Input: part model. Units: mm. Frame: model coordinates. A direction names the side the tool comes from. Coordinates: 2 decimals unless noted, no trailing zeros. Loops run counter-clockwise (first coordinate to the right, second up) from the corner with the lowest first, then second, coordinate; pieces in that order, holes last.
```python
from build123d import *

# Parameters (mm, degrees)
SKETCH1_W           = 350
SKETCH1_H           = 150
BOSS_EXTRUDE1_DEPTH = 10
SKETCH2_W           = 328
SKETCH2_H           = 126
SKETCH2_W_2         = 70
SKETCH2_H_2         = 110
SKETCH2_W_3         = 27.5
SKETCH2_H_3         = 55
CUT_EXTRUDE1_DEPTH  = 9.5


with BuildPart() as part:
    # Sketch1 → Boss-Extrude1 (new body)
    with BuildSketch(Plane(origin=(0, 0, 0), x_dir=(1, 0, 0), z_dir=(0, 1, 0))):
        Rectangle(SKETCH1_W, SKETCH1_H)
    extrude(amount=BOSS_EXTRUDE1_DEPTH)

    # Sketch2 → Cut-Extrude1 (cut)
    # profile 1 of 5: a face of its own
    with BuildSketch(Plane(origin=(0, 10, 0), x_dir=(1, 0, 0), z_dir=(0, 1, 0))):
        with Locations((-1, -2)):
            Rectangle(SKETCH2_W, SKETCH2_H)
        with Locations((-122, -2)):
            Rectangle(SKETCH2_W_2, SKETCH2_H_2, mode=Mode.SUBTRACT)
        with Locations((-41, -2)):
            Rectangle(SKETCH2_W_2, SKETCH2_H_2, mode=Mode.SUBTRACT)
        with Locations((40, -2)):
            Rectangle(SKETCH2_W_2, SKETCH2_H_2, mode=Mode.SUBTRACT)
        with Locations((121, -2)):
            Rectangle(SKETCH2_W_2, SKETCH2_H_2, mode=Mode.SUBTRACT)
    # profile 2 of 5: a face of its own
    with BuildSketch(Plane(origin=(0, 10, 0), x_dir=(1, 0, 0), z_dir=(0, 1, 0))):
        with BuildLine():
            Line((-147, -44.243757332), (-147, 40.243757332))
            ThreePointArc((-147, 40.243757332), (-147.353553391, 43.353553391), (-144.243757332, 43))
            Line((-144.243757332, 43), (-99.756242668, 43))
            ThreePointArc((-99.756242668, 43), (-96.646446609, 43.353553391), (-97, 40.243757332))
            Line((-97, 40.243757332), (-97, -44.243757332))
            ThreePointArc((-97, -44.243757332), (-96.646446609, -47.353553391), (-99.756242668, -47))
            Line((-99.756242668, -47), (-144.243757332, -47))
            ThreePointArc((-144.243757332, -47), (-147.353553391, -47.353553391), (-147, -44.243757332))
        make_face()
        with Locations((-121.25, -3.5)):
            Rectangle(SKETCH2_W_3, SKETCH2_H_3, mode=Mode.SUBTRACT)
    # profile 3 of 5: a face of its own
    with BuildSketch(Plane(origin=(0, 10, 0), x_dir=(1, 0, 0), z_dir=(0, 1, 0))):
        with BuildLine():
            Line((-66, -44.243757332), (-66, 40.243757332))
            ThreePointArc((-66, 40.243757332), (-66.353553391, 43.353553391), (-63.243757332, 43))
            Line((-63.243757332, 43), (-18.756242668, 43))
            ThreePointArc((-18.756242668, 43), (-15.646446609, 43.353553391), (-16, 40.243757332))
            Line((-16, 40.243757332), (-16, -44.243757332))
            ThreePointArc((-16, -44.243757332), (-15.646446609, -47.353553391), (-18.756242668, -47))
            Line((-18.756242668, -47), (-63.243757332, -47))
            ThreePointArc((-63.243757332, -47), (-66.353553391, -47.353553391), (-66, -44.243757332))
        make_face()
        with Locations((-40.25, -3.5)):
            Rectangle(SKETCH2_W_3, SKETCH2_H_3, mode=Mode.SUBTRACT)
    # profile 4 of 5: a face of its own
    with BuildSketch(Plane(origin=(0, 10, 0), x_dir=(1, 0, 0), z_dir=(0, 1, 0))):
        with BuildLine():
            Line((15, -44.243757332), (15, 40.243757332))
            ThreePointArc((15, 40.243757332), (14.646446609, 43.353553391), (17.756242668, 43))
            Line((17.756242668, 43), (62.243757332, 43))
            ThreePointArc((62.243757332, 43), (65.353553391, 43.353553391), (65, 40.243757332))
            Line((65, 40.243757332), (65, -44.243757332))
            ThreePointArc((65, -44.243757332), (65.353553391, -47.353553391), (62.243757332, -47))
            Line((62.243757332, -47), (17.756242668, -47))
            ThreePointArc((17.756242668, -47), (14.646446609, -47.353553391), (15, -44.243757332))
        make_face()
        with Locations((40.75, -3.5)):
            Rectangle(SKETCH2_W_3, SKETCH2_H_3, mode=Mode.SUBTRACT)
    # profile 5 of 5: a face of its own
    with BuildSketch(Plane(origin=(0, 10, 0), x_dir=(1, 0, 0), z_dir=(0, 1, 0))):
        with BuildLine():
            Line((98.756242668, -47), (143.243757332, -47))
            ThreePointArc((143.243757332, -47), (146.353553391, -47.353553391), (146, -44.243757332))
            Line((146, -44.243757332), (146, 40.243757332))
            ThreePointArc((146, 40.243757332), (146.353553391, 43.353553391), (143.243757332, 43))
            Line((143.243757332, 43), (98.756242668, 43))
            ThreePointArc((98.756242668, 43), (95.646446609, 43.353553391), (96, 40.243757332))
            Line((96, 40.243757332), (96, -44.243757332))
            ThreePointArc((96, -44.243757332), (95.646446609, -47.353553391), (98.756242668, -47))
        make_face()
        with Locations((121.75, -3.5)):
            Rectangle(SKETCH2_W_3, SKETCH2_H_3, mode=Mode.SUBTRACT)
    extrude(amount=-CUT_EXTRUDE1_DEPTH, mode=Mode.SUBTRACT)


solid = part.part
```
Item 1: Section query B-B (y = 2.75). Count the separate pieces of the cut face and the enclosed holes in it, then the cut area to 3 significant figures.
Result:
separate pieces: 9
enclosed holes: 5
area: 30,000 mm2
Item 2: Section query D-D (x = -139). Output: boundary loops of the cut face in (y, z), then the cut area to 3 significant figures.
Result:
outline: (0, -75) - (10, -75) - (10, -61) - (0.5, -61) - (0.5, -53) - (10, -53) - (10, -43) - (0.5, -43) - (0.5, 47) - (10, 47) - (10, 57) - (0.5, 57) - (0.5, 65) - (10, 65) - (10, 75) - (0, 75) - close
area: 493 mm2
Item 3: Mould query, pull axis Z, two halves, no side actions, for faces 3 (the face through (-121, 10, 3)), 4 (the face through (-135, 5, 4)). Classes: +Z half, -Z half, draft (parallel to the pull), parting line (faces both ways), or undercut.
Result:
face 3: draft
face 4: undercut
Item 4: Section query C-C (x = -1). Output: boundary loops of the cut face in (y, z).
Result:
outline: (0, -75) - (10, -75) - (10, -61) - (0.5, -61) - (0.5, 65) - (10, 65) - (10, 75) - (0, 75) - close
Item 5: Line query: L1, parallel to Z at x = 8, y = 5.75; L2, parallel to Z at x = 132.5, y = 5; L3, parallel to X at y = 3, z = -46.5. Output: solid intervals per line, ascending.
Result:
L1: z = -75 to -61, -53 to 57, 65 to 75
L2: z = -75 to -61, -53 to -43, -24 to 31, 47 to 57, 65 to 75
L3: x = -175 to -165, -157 to -87, -76 to -6, 5 to 75, 86 to 156, 163 to 175
Item 6: Reachability of faces 1 (the face through (-107.5, 5, 4)), 2 (the face through (-40, 10, 3)) from +Z, -Z, +X, -X, +Y, -Y: full face, straight path, thin tool, end or side. Return the list, or none.
Result:
face 1: +Y
face 2: +Z, -Z, +X, -X, +Y
Item 7: Contact query for a flat-ended pin moving along its axis: P1, Ø3, axis at x = 63.94, z = 45.94, coming from the +Y side. Output: stop coordinate, or through.
Result:
P1: stops at y = 0.5
Item 8: Section query A-A (z = 52.5). Output: boundary loops of the cut face in (x, y).
Result:
outline: (-175, 0) - (175, 0) - (175, 10) - (163, 10) - (163, 0.5) - (156, 0.5) - (156, 10) - (86, 10) - (86, 0.5) - (75, 0.5) - (75, 10) - (5, 10) - (5, 0.5) - (-6, 0.5) - (-6, 10) - (-76, 10) - (-76, 0.5) - (-87, 0.5) - (-87, 10) - (-157, 10) - (-157, 0.5) - (-165, 0.5) - (-165, 10) - (-175, 10) - close
